```python
from build123d import *

# Parameters (mm, degrees)
F0_W     = 76.2
F0_H     = 50.8
F0_R     = 12.7
F1_DEPTH = 12.7
F2_W     = 6.35
F2_H     = 50.8
F3_DEPTH = 2.54


with BuildPart() as f1:
    # F0 (on Top) → F1 (new body)
    with BuildSketch(Plane.XY):
        Rectangle(F0_W, F0_H)
        Circle(F0_R, mode=Mode.SUBTRACT)
    extrude(amount=F1_DEPTH)

    # F2 (on face) → F3 (cut)
    with BuildSketch(Plane.XY.offset(12.7)):
        with Locations((-32.385, 0)):
            Rectangle(F2_W, F2_H)
        with BuildLine():
            Line((6.35, 25.4), (-6.35, 25.4))
            Line((-6.35, 25.4), (-6.35, 10.9985226281))
            ThreePointArc((-6.35, 10.9985226281), (0, 12.7), (6.35, 10.9985226281))
            Line((6.35, 10.9985226281), (6.35, 25.4))
        make_face()
        with BuildLine():
            Line((-6.35, -10.9985226281), (-6.35, -25.4))
            Line((-6.35, -25.4), (6.35, -25.4))
            Line((6.35, -25.4), (6.35, -10.9985226281))
            ThreePointArc((6.35, -10.9985226281), (0, -12.7), (-6.35, -10.9985226281))
        make_face()
    extrude(amount=-F3_DEPTH, mode=Mode.SUBTRACT)


solid = f1.part
```
Geometry: final body of the model. Coordinates: model frame, mm. A direction names the side the tool comes from. Coordinates: 2 decimals unless noted, no trailing zeros. Order: outer loops, then holes, each group sorted by start corner. A loop starts at its lowest first (then second) coordinate and runs counter-clockwise, first axis right, second up. Notation, with made-up numbers: M 44,43.5 L 49,43.5 A16 ccw 49,69.5 Z; hole C 74,14.25 d6. An arc over 180 degrees is marked long. Answer in a Markdown table with one row per item. Add a question column.
Q1. Section query C-C on x = 0. Return the cut outline in (y, z).
Q2. Section query A-A on y = 0. Return the cut outline in (x, z).
Q3. Reachability of faces 1 (the flat face through (-35.56, 0, 11)), 2 (the flat face through (22, 0, 12.7)) from +Z, -Z, +X, -X, +Y, -Y: full face, straight path, thin tool, end or side. Return the list, or none.
Q4. Mould query, pull axis Y, two halves, no side actions, for faces 3 (the flat face through (-1, -25.4, 6)), 4 (the flat face through (-32, 0, 10.16)), 5 (the cylindrical face through (-1.653, 12.592, 6.261)). Classes: released by +Y, released by -Y, zero draft, split by the parting line, or undercut.
Q5. Section query B-B on z = 7.25. Return the cut outline in (x, y), and give its area (3 significant figures).
Q6. Section query D-D on y = 13.5. Return the cut outline in (x, z).
Q7. Line query: L1, parallel to X at y = -20.5, z = 10.5; L2, parallel to Y at x = 0, z = 3.75; L3, parallel to X at y = 0, z = 7.75. Output: solid intervals per line, ascending.
Q8. Contact query for flat-ended pins moving along their axis: P1, Ø10, axis at x = -1.5, y = 20.5, coming from the +Z side; P2, Ø1.9, axis at x = -32.5, y = 1.5, coming from the +Z side. Output: stop coordinate, or through.
Completed:
| question | item | result |
|---|---|---|
| 1 | outline | M -25.4,0 L -12.7,0 L -12.7,10.16 L -25.4,10.16 Z; M 12.7,0 L 25.4,0 L 25.4,10.16 L 12.7,10.16 Z |
| 2 | outline | M -38.1,0 L -12.7,0 L -12.7,12.7 L -29.21,12.7 L -29.21,10.16 L -35.56,10.16 L -35.56,12.7 L -38.1,12.7 Z; M 12.7,0 L 38.1,0 L 38.1,12.7 L 12.7,12.7 Z |
| 3 | face 1 | +Z, +Y, -Y |
| 3 | face 2 | +Z, +X, -X, +Y, -Y |
| 4 | face 3 | released by -Y |
| 4 | face 4 | zero draft |
| 4 | face 5 | undercut |
| 5 | outline | M -38.1,-25.4 L 38.1,-25.4 L 38.1,25.4 L -38.1,25.4 Z; hole C 0,0 d25.4 |
| 5 | area | 3,360 mm2 |
| 6 | outline | M -38.1,0 L 38.1,0 L 38.1,12.7 L 6.35,12.7 L 6.35,10.16 L -6.35,10.16 L -6.35,12.7 L -29.21,12.7 L -29.21,10.16 L -35.56,10.16 L -35.56,12.7 L -38.1,12.7 Z |
| 7 | L1 | x = -38.1 to -35.56, -29.21 to -6.35, 6.35 to 38.1 |
| 7 | L2 | y = -25.4 to -12.7, 12.7 to 25.4 |
| 7 | L3 | x = -38.1 to -12.7, 12.7 to 38.1 |
| 8 | P1 | stops at z = 12.7 |
| 8 | P2 | stops at z = 10.16 |
